from build123d import *

# Parameters (mm, degrees)
SKETCH_2_W = 370
SKETCH_2_H = 1


with BuildPart() as part:
    # 扫描1: sweep along a path in 草图1
    with BuildLine(Plane(origin=(0, 0, -202.897842698), x_dir=(-1, 0, 0), z_dir=(0, 0, -1))) as sweep_1_path:
        Line((80.56049666, 160.574025873), (780.56049666, 160.574025873))
        ThreePointArc((780.56049666, 160.574025873), (805.56049666, 135.574025873), (780.56049666, 110.574025873))
        Line((780.56049666, 110.574025873), (80.56049666, 110.574025873))
        ThreePointArc((80.56049666, 110.574025873), (55.56049666, 135.574025873), (80.56049666, 160.574025873))
    # 草图2 → 扫描1 (sweep)
    with BuildSketch(Plane(origin=(-80.56049666, 0, 0), x_dir=(0, 0, -1), z_dir=(1, 0, 0))):
        with Locations((17.897842698, 161.5)):
            Rectangle(SKETCH_2_W, SKETCH_2_H)
    sweep(path=sweep_1_path.line)


solid = part.part
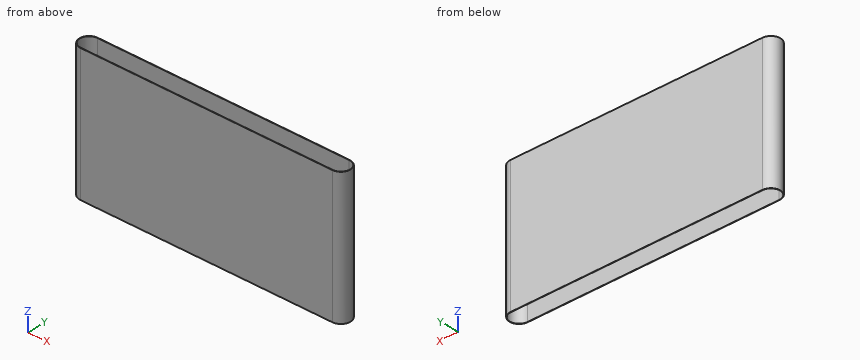
Geometry: final body of the model. Coordinates: model frame, mm. Give positions to 0.01 mm unless a question says otherwise; leave off trailing zeros. Write each loop counter-clockwise with the first axis right and the second up, starting at its lowest first coordinate (ties: lowest second). Pieces come first, ordered by that corner, then holes.
(1) Cut plane B-B, the plane y = 124.5. Return loops of the section in (x, z).
(2) Cut plane C-C, the plane z = 116. Return loops of the section in (x, y), then the cut area to 3 significant figures.
(3) Ray query, line 1 (Y direction, x = -558.5, z = -123); line 2 (X direction, y = 159, z = 131); line 3 (X direction, y = 158, z = 116). Return the intervals inside material, ascending.
(4) Cut plane A-A, the plane x = -183. Return loops of the section in (y, z), then the cut area to 3 significant figures.
(5) First-contact query: P1, Ø1, axis at y = 114.5, z = 95, coming from the -X side; P2, Ø12, axis at y = 154, z = -80.5, coming from the -X side. Flat tips, straight axial feed; report the tip coordinate or a pass-through.
Values follow:
1. outline: (-804.55, -202.9) - (-803.45, -202.9) - (-803.45, 167.1) - (-804.55, 167.1) - close; (-57.67, -202.9) - (-56.57, -202.9) - (-56.57, 167.1) - (-57.67, 167.1) - close
2. outline: (-780.56, 109.15) - (-80.56, 109.15) arc R26.43 ccw to (-80.56, 162) - (-780.56, 162) arc R26.43 ccw to start; hole (-780.56, 110.15) - (-80.56, 110.15) arc R25.43 ccw to (-80.56, 161) - (-780.56, 161) arc R25.43 ccw to start
2. area: 1,560 mm2
3. line 1: y = 109.15 to 110.15, 161 to 162
3. line 2: x = -792.79 to -790.45, -70.68 to -68.33
3. line 3: x = -794.54 to -792.54, -68.58 to -66.58
4. outline: (109.15, -202.9) - (110.15, -202.9) - (110.15, 167.1) - (109.15, 167.1) - close; (161, -202.9) - (162, -202.9) - (162, 167.1) - (161, 167.1) - close
4. area: 740 mm2
5. P1: stops at x = -797.14
5. P2: stops at x = -803.88
